Could you check a few things on this model? Use its own coordinates, in mm. Give positions to 0.01 mm unless a question says otherwise; leave off trailing zeros. Loops run counter-clockwise (first coordinate to the right, second up) from the corner with the lowest first, then second, coordinate; pieces in that order, holes last.
1. I need wall thicknesses on line 1 along Z through (x, y) = (-1.65, 38); line 2 along Y through (x, z) = (1.25, 0); line 3 along Z through (x, y) = (-1.4, -38). Which ranges of each line are inside material? Lowest first, please.
2. Imagine slicing it at A-A (z = 25). List the corners of the cut face in (x, y) for me.
3. For P1, Ø5.5, axis at y = -38, z = 0, coming from the +X side; P2, Ø2.5, axis at y = 12, z = 0, coming from the -X side, each with a flat end and sliding along its axis, tell me the tip position at first contact or that it passes through.
4. Imagine slicing it at C-C (y = -27.5). List the corners of the cut face in (x, z) for me.
5. Imagine slicing it at B-B (y = 12). List the corners of the cut face in (x, z) for me, plus the area to 3 significant figures.
Autodesk Inventor part; units mm, degrees
ref_plane "YZ Plane" through (0, 0, 0) normal (1, 0, 0) x (0, 1, 0)
ref_plane "XZ Plane" through (0, 0, 0) normal (0, 1, 0) x (-1, 0, 0)
ref_plane "XY Plane" through (0, 0, 0) normal (0, 0, 1) x (1, 0, 0)
sketch "Skizze1" plane through (0, 0, 0) normal (1, 0, 0) x (0, 1, 0)
  line L0 (-63, 0) -> (63, 0)
  line L1 (0, 42) -> (0, -42)
  line L2 (-45, 30) -> (45, 30)
  line L3 (45, 30) -> (45, -30)
  line L4 (45, -30) -> (-45, -30)
  line L5 (-45, -30) -> (-45, 30)
  line L6 (-45, 30) -> (45, -30) construction
  line L7 (45, 30) -> (-45, -30) construction
  point P0 (0, 0)
  dimension "d21" = 90
  dimension "d22" = 60
extrude "Extrusion1" add sketch "Skizze1" along normal mid plane 5
sketch "Skizze2" plane through (2.5, 0, 0) normal (1, 0, 0) x (0, 0, -1)
  line L0 (-42, 0) -> (42, 0)
  line L1 (0, -63) -> (0, 63)
  line L2 (-30, -45) -> (30, -45)
  point P0 (0, 0)
  point P1 (0, 12)
  point P2 (0, -38)
  dimension "d23" = 50
  dimension "d24" = 7
hole "Bohrung1" at (2.5, -38, 0) at (2.5, 12, 0) direction (-1, 0, 0) diameter 3.4 end through all counterbore diameter 6.5 counterbore depth 3.4
sketch "Skizze3" plane through (2.5, 0, 0) normal (1, 0, 0) x (0, 0, -1)
  line L0 (0, -63) -> (0, 63)
  line L1 (-42, 0) -> (42, 0)
  line L2 (-25, -40) -> (-25, 40) construction
  line L3 (-23.35, -40) -> (-23.35, 40)
  line L4 (-26.65, 40) -> (-26.65, -40)
  arc A0 (-26.65, -40) -> (-23.35, -40) centre (-25, -40) ccw
  arc A1 (-23.35, 40) -> (-26.65, 40) centre (-25, 40) ccw
  point P0 (0, 0)
  point P1 (-25, 0)
  point P2 (-26.65, 0)
  point P3 (-23.35, 0)
  dimension "d14" = 3.3
  dimension "d15" = 80
  dimension "d16" = 25
extrude "Extrusion2" cut sketch "Skizze3" against normal through all
mirror "Spiegeln1" about plane through (0, 0, 0) normal (0, 0, 1) of "Extrusion2"
fillet "Rundung1" radius 4 4 edges at (0, 45, 30) (0, 45, -30) (0, -45, 30) (0, -45, -30)
properties part number "24_Laserholder" material "PET-Kunststoff"
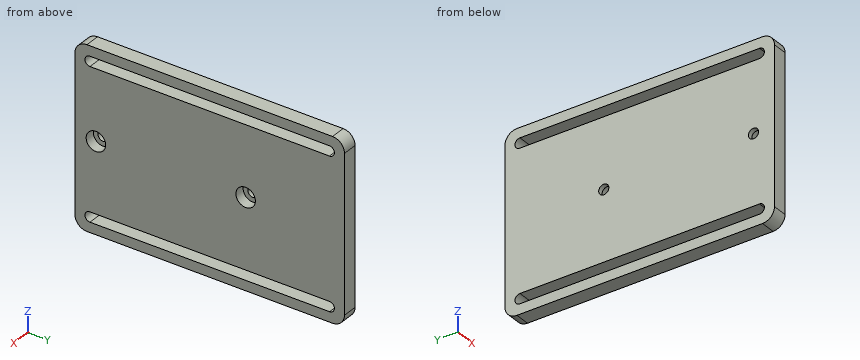
Derived:
1. line 1: z = -30 to -26.65, -23.35 to 23.35, 26.65 to 30
1. line 2: y = -45 to -41.25, -34.75 to 8.75, 15.25 to 45
1. line 3: z = -30 to -26.65, -23.35 to -1.7, 1.7 to 23.35, 26.65 to 30
2. outline: (-2.5, -45) - (2.5, -45) - (2.5, -41.65) - (-2.5, -41.65) - close; (-2.5, 41.65) - (2.5, 41.65) - (2.5, 45) - (-2.5, 45) - close
3. P1: stops at x = -0.9
3. P2: passes through
4. outline: (-2.5, -30) - (2.5, -30) - (2.5, -26.65) - (-2.5, -26.65) - close; (-2.5, -23.35) - (2.5, -23.35) - (2.5, 23.35) - (-2.5, 23.35) - close; (-2.5, 26.65) - (2.5, 26.65) - (2.5, 30) - (-2.5, 30) - close
5. outline: (-2.5, -30) - (2.5, -30) - (2.5, -26.65) - (-2.5, -26.65) - close; (-2.5, -23.35) - (2.5, -23.35) - (2.5, -3.25) - (-0.9, -3.25) - (-0.9, -1.7) - (-2.5, -1.7) - close; (-2.5, 1.7) - (-0.9, 1.7) - (-0.9, 3.25) - (2.5, 3.25) - (2.5, 23.35) - (-2.5, 23.35) - close; (-2.5, 26.65) - (2.5, 26.65) - (2.5, 30) - (-2.5, 30) - close
5. area: 239 mm2
